from build123d import *

# Parameters (mm, degrees)
BOSS_EXTRUDE1_DEPTH        = 3.2893
FILLET1_R                  = 3.175
F_97_0_26_DIAMETER_HOLE1_D = 6.604


with BuildPart() as part:
    # Sketch1 → Boss-Extrude1 (new, symmetric)
    with BuildSketch(Plane.XY):
        with BuildLine():
            Line((26.092747392, -18.613926775), (9.438661748, -30.801947025))
            Line((9.438661748, -30.801947025), (9.438661748, -42.398036845))
            Line((9.438661748, -42.398036845), (55.450257601, -42.398036845))
            Line((55.450257601, -42.398036845), (55.450257601, 40.151963155))
            Line((55.450257601, 40.151963155), (-8.049742399, 40.151963155))
            Line((-8.049742399, 40.151963155), (-8.049742399, 30.753963155))
            ThreePointArc((-8.049742399, 30.753963155), (-1.129436116, 25.949070048), (2.010067235, 18.131068031))
            ThreePointArc((2.010067235, 18.131068031), (2.969578149, 13.959464366), (5.008768553, 10.19587023))
            Line((5.008768553, 10.19587023), (26.092747392, -18.613926775))
        make_face()
    extrude(amount=BOSS_EXTRUDE1_DEPTH, both=True)

    # Fillet1
    fillet1_edges = [part.edges().sort_by_distance(p)[0] for p in [
        (26.092747392, -18.613926775, 0),
    ]]
    fillet(fillet1_edges, radius=FILLET1_R)

    # #97 (0.26) Diameter Hole1 (through all)
    with Locations(Plane(origin=(42.750257601, 27.451963155, 3.2893), x_dir=(1, 0, 0), z_dir=(0, 0, 1))):
        with Locations((0, 0), (0, -57.15)):
            Hole(F_97_0_26_DIAMETER_HOLE1_D / 2)


solid = part.part
Verification items for the finished model (mm, model axes). A direction names the side the tool comes from. Round coordinates to 2 decimals unless told otherwise and drop trailing zeros. Loops run counter-clockwise (first coordinate to the right, second up) from the corner with the lowest first, then second, coordinate; pieces in that order, holes last. Notation, with made-up numbers: (-17, 27) - (21, 27) arc R20 ccw to (21, 59) - close; hole circle Ø8 at (64.5, 16). An arc over 180 degrees is marked (long way). Use a Markdown table: item, result. Add a question column.
1. Section check A-A, the plane x = 20.5. Record the boundary of the cut face in (y, z), plus the area to 3 significant figures.
2. Release check for a two-part mould opening along X. For faces 1 (the face through (39.7, -30.96, -0.05)), 2 (the face through (24, 40.152, 0)), 3 (the face through (39.7, 26.19, -0.05)), 4 (the face through (2.948, 14.016, 0.046)) record: released by +X, released by -X, zero draft, split by the parting line, or undercut.
3. Section check C-C, the plane y = -34. Record the boundary of the cut face in (x, z), plus the area to 3 significant figures.
4. Thickness scan on probe 1 along Y at (x, z) = (45, -2.5); probe 2 along Y at (x, z) = (41, 2.5); probe 3 along Y at (x, z) = (11, 1). Record the ranges inside material, lowest first. Write a range as [from, to].
5. Section check B-B, the plane z = -0.5. Give the number of separate pieces and of enclosed holes in the cut face, plus the area to 3 significant figures.
6. Access from +Z, -Z, +X, -X, +Y, -Y to the whole of each face (thin tool, end or side, straight path). Record for faces 5 (the face through (14.479, -2.744, 0.046)), 6 (the face through (55.45, -2, 0)), 7 (the face through (9.439, -37, 0)).
7. Section check D-D, the plane y = -3.5. Record the boundary of the cut face in (x, z).
8. Gauge pin test, flat ends, axial feed: pin 1 (4 mm diameter, centred on x = 42.75, y = 27.45, fed in from +Z); pin 2 (1 mm diameter, centred on y = 18, z = 0.5, fed in from -X). Record the tip position at first contact, or that the pin passes through.
Checks:
| question | item | result |
|---|---|---|
| 1 | outline | (-42.4, -3.29) - (-22.71, -3.29) - (-22.71, 3.29) - (-42.4, 3.29) - close; (-10.97, -3.29) - (40.15, -3.29) - (40.15, 3.29) - (-10.97, 3.29) - close |
| 1 | area | 466 mm^2 |
| 2 | face 1 | undercut |
| 2 | face 2 | zero draft |
| 2 | face 3 | undercut |
| 2 | face 4 | released by -X |
| 3 | outline | (9.44, -3.29) - (55.45, -3.29) - (55.45, 3.29) - (9.44, 3.29) - close |
| 3 | area | 303 mm^2 |
| 4 | probe 1 | y = [-42.4, -32.12], [-27.28, 25.03], [29.87, 40.15] |
| 4 | probe 2 | y = [-42.4, -32.5], [-26.9, 24.65], [30.25, 40.15] |
| 4 | probe 3 | y = [-42.4, -29.66], [2.01, 40.15] |
| 5 | separate pieces | 1 |
| 5 | enclosed holes | 2 |
| 5 | area | 3,800 mm^2 |
| 6 | face 5 | +Z, -Z, -X |
| 6 | face 6 | +Z, -Z, +X, +Y, -Y |
| 6 | face 7 | +Z, -Z, -X, -Y |
| 7 | outline | (15.03, -3.29) - (55.45, -3.29) - (55.45, 3.29) - (15.03, 3.29) - close |
| 8 | pin 1 | passes through |
| 8 | pin 2 | stops at x = 1.97 |
